Check sheet for the modelled part. Datum: model origin and axes. Units: mm. A direction names the side the tool comes from. Round coordinates to 2 decimals unless told otherwise and drop trailing zeros. Loops run counter-clockwise (first coordinate to the right, second up) from the corner with the lowest first, then second, coordinate; pieces in that order, holes last. Notation, with made-up numbers: (84.5, 77) - (96.5, 77) arc R25 ccw to (96.5, 107) - close; hole circle Ø6 at (-12.75, 2.25). An arc over 180 degrees is marked (long way). Put each result on its own line as item: value.
Autodesk Inventor part; units mm, degrees
ref_plane "YZ Plane" through (0, 0, 0) normal (1, 0, 0) x (0, 1, 0)
ref_plane "XZ Plane" through (0, 0, 0) normal (0, 1, 0) x (-1, 0, 0)
ref_plane "XY Plane" through (0, 0, 0) normal (0, 0, 1) x (1, 0, 0)
sketch "Skizze1" plane through (0, 0, 0) normal (0, 0, 1) x (1, 0, 0)
  line L0 (-49, 0) -> (49, 0) construction
  circle A0 centre (0, 0) radius 35
  line L1 (-10, 28) -> (10, 28)
  line L2 (10, 28) -> (10, 25)
  line L3 (10, 25) -> (-10, 25)
  line L4 (-10, 25) -> (-10, 28)
  line L5 (1.5, 25) -> (-1.5, 25)
  line L6 (-1.5, 25) -> (-1.5, 20)
  line L7 (-1.5, 20) -> (1.5, 20)
  line L8 (1.5, 20) -> (1.5, 25)
  circle A1 centre (0, 0) radius 4.5
  line L9 (0, 49) -> (0, -49) construction
  dimension "d9" = 70
  dimension "d10" = 3
  dimension "d11" = 25
  dimension "d14" = 20
  dimension "d23" = 5
  dimension "d62" = 9
extrude "Extrusion3" add sketch "Skizze1" against normal blind 7 contours L1 L2 L3 L4 | L3 L8 L7 L6
fillet "Rundung1" radius 4 2 edges at (-10, 26.5, -7) (10, 26.5, -7)
sketch "Skizze2" plane through (-10, 28, 0) normal (0, 1, 0) x (1, 0, 0)
  circle A0 centre (3, 4) radius 1.1
  circle A1 centre (17, 4) radius 1.1
  line L0 (10, 0) -> (10, 7) construction
  line L1 (43, 0) -> (-27, 0) construction
  line L2 (-1.6221, 4) -> (19.0112, 4) construction
  line L3 (4, 7) -> (16, 7) construction
  line L4 (0, 0) -> (0, 3)
  dimension "d16" = 2.2
  dimension "d20" = 3
  dimension "d21" = 3
extrude "Extrusion4" cut sketch "Skizze2" against normal up to next
chamfer "Fase1" distance 5 distance2 7 1 edges at (0, 20, -7) measured on face at (0.5, 27, -7)
pattern_circular "Runde Anordnung1" count 3 over 360 about axis through (0, 0, -10) along (0, 0, 1) of "Extrusion3", "Extrusion4", "Fase1", "Rundung1"
extrude "Extrusion11" add sketch "Skizze1" along normal blind 2 contours A0 | L1 L2 L3 L4 | L3 L8 L7 L6
fillet "Rundung5" radius 1 4 edges at (-35, 0, 2) (-4.5, 0, 2) (-4.5, 0, 0) (-35, 0, 0)
equation "\"d21\" = d20"
properties part number "Stewart-Sym-Base"
Item 1: Section check B-B on z = -6. Enter the section's corners in (x, y), then the cut area to 3 significant figures.
Filled sheet:
outline: (-28.57, -6.51) - (-19.93, -21.49) - (-17.33, -19.99) - (-20.9, -13.8) - (-20.28, -13.44) - (-21.78, -10.84) - (-22.4, -11.2) - (-25.97, -5.01) - close; (-8.65, 25) - (-1.5, 25) - (-1.5, 24.29) - (1.5, 24.29) - (1.5, 25) - (8.65, 25) - (8.65, 28) - (-8.65, 28) - close; (17.33, -19.99) - (19.93, -21.49) - (28.57, -6.51) - (25.97, -5.01) - (22.4, -11.2) - (21.78, -10.84) - (20.28, -13.44) - (20.9, -13.8) - close
area: 162 mm²
Item 2: Tool access check on faces 5 (the flat face through (24.496, -7.572, -3.451)), 6 (the flat face through (-18.805, -17.428, -3.451)), 7 (the flat face through (27.93, -4.58, -1.48)), 8 (the flat face through (-17.93, -21.9, -1.48)). Record the directions out of +Z, -Z, +X, -X, +Y, -Y that give a thin tool (end or side, any length) a straight path to the whole face; none if there is none.
Filled sheet:
face 5: -Z, +Y
face 6: -Z
face 7: -Z, +X, +Y
face 8: -Z, -Y
Item 3: Release check for a two-part mould opening along X. For faces 1 (the flat face through (1.5, 23, -3)), 2 (the cylindrical face through (-27.33, -5.62, -5.86)), 3 (the flat face through (18.746, -17.531, -3.451)), 4 (the flat face through (0, 22.5, -3.5)) record: +X half, -X half, draft (parallel to the pull), parting line (faces both ways), or undercut.
Filled sheet:
face 1: +X half
face 2: -X half
face 3: undercut
face 4: draft
Item 4: Go/stop test with flat-tipped pins: pin 1 (0.9 mm diameter, centred on y = 26.5, z = -1.5, fed in from -X); pin 2 (5 mm diameter, centred on x = 7.5, z = -4, fed in from -Y); pin 3 (5 mm diameter, centred on y = -6, z = -3.5, fed in from +X); pin 4 (10 mm diameter, centred on x = -25.5, y = -7, fed in from -Z). Record where each tip stops, or that it passes through.
Filled sheet:
pin 1: x = -10
pin 2: y = 25
pin 3: x = 29.25
pin 4: z = -7
Item 5: Thickness scan on line 1 (Y direction, x = 0, z = 1); line 2 (X direction, y = 26.55, z = -4); line 3 (Z direction, x = 19.5, y = -15). Record the ranges inside material, lowest first. Write a range as from..to.
Filled sheet:
line 1: -35..-4.5, 4.5..35
line 2: -9.87..-8.1, -5.9..5.9, 8.1..9.87
line 3: 0..2
